Design review of the part built by this model. Coordinates are the model's own, in mm. A direction names the side the tool comes from. Give positions to 0.01 mm unless a question says otherwise; leave off trailing zeros. Write each loop counter-clockwise with the first axis right and the second up, starting at its lowest first coordinate (ties: lowest second). Pieces come first, ordered by that corner, then holes.
```python
from build123d import *

# Parameters (mm, degrees)
F0_W      = 400
F0_H      = 500
F1_DEPTH  = 2
F2_W      = 400
F2_H      = 500
F2_W_2    = 396
F2_H_2    = 496
F3_DEPTH  = 248
F5_DEPTH  = 500
F7_DEPTH  = 20
F8_R      = 5
F10_R     = 4
F11_DEPTH = 25
F12_R     = 5


with BuildPart() as f1:
    # F0 (on Top) → F1 (new body)
    with BuildSketch(Plane.XY):
        Rectangle(F0_W, F0_H)
    extrude(amount=F1_DEPTH)

    # F2 (on face) → F3 (join)
    with BuildSketch(Plane.XY.offset(2)):
        Rectangle(F2_W, F2_H)
        Rectangle(F2_W_2, F2_H_2, mode=Mode.SUBTRACT)
    extrude(amount=F3_DEPTH)

    # F4 (on face) → F5 (join)
    with BuildSketch(Plane.XZ.offset(250)):
        Polygon((215, 250), (200, 250), (200, 235), (202, 235), (202, 248), (215, 248), align=None)
        Polygon((-200, 235), (-200, 250), (-215, 250), (-215, 248), (-202, 248), (-202, 235), align=None)
    extrude(amount=-F5_DEPTH)

    # F6 (on Right) → F7 (join, symmetric)
    with BuildSketch(Plane.YZ):
        with BuildLine():
            Line((-256, 260), (-280, 260))
            Line((-280, 260), (-280, 256))
            Line((-280, 256), (-256, 256))
            ThreePointArc((-256, 256), (-254.585786, 255.414214), (-254, 254))
            Line((-254, 254), (-254, 230))
            Line((-254, 230), (-250, 230))
            Line((-250, 230), (-250, 254))
            ThreePointArc((-250, 254), (-251.757359, 258.242641), (-256, 260))
        make_face()
    extrude(amount=F7_DEPTH, both=True)

    # F8
    f8_edges = [f1.edges().sort_by_distance(p)[0] for p in [
        (20, -280, 258),
        (-20, -280, 258),
    ]]
    fillet(f8_edges, radius=F8_R)

    # F10 (on face) → F11 (cut)
    with BuildSketch(Plane.XY.offset(260)):
        with Locations((0, -270)):
            Circle(F10_R)
    extrude(amount=-F11_DEPTH, mode=Mode.SUBTRACT)

    # F12
    f12_edges = [f1.edges().sort_by_distance(p)[0] for p in [
        (20, -252, 230),
        (-20, -252, 230),
    ]]
    fillet(f12_edges, radius=F12_R)


solid = f1.part
```
(1) Consider section C-C, the plane x = 47. Give the boundary of the cut face in (y, z), then the cut area to 3 significant figures.
Resolved:
outline: (-250, 0) - (250, 0) - (250, 250) - (248, 250) - (248, 2) - (-248, 2) - (-248, 250) - (-250, 250) - close
area: 1,990 mm2
(2) Consider section A-A, the plane z = 98. Give the boundary of the cut face in (x, y).
Resolved:
outline: (-200, -250) - (200, -250) - (200, 250) - (-200, 250) - close; hole (-198, -248) - (198, -248) - (198, 248) - (-198, 248) - close
(3) To check wall thickness, follow L1, parallel to X at y = 111.5, z = 230; L2, parallel to X at y = 184, z = 239; L3, parallel to Y at x = 16, z = 43. State the ranges of each line that lie inside material, in increasing order.
Resolved:
L1: x = -200 to -198, 198 to 200
L2: x = -202 to -198, 198 to 202
L3: y = -250 to -248, 248 to 250
(4) Consider section B-B, the plane y = -165. Give the boundary of the cut face in (x, z).
Resolved:
outline: (-215, 248) - (-202, 248) - (-202, 235) - (-200, 235) - (-200, 0) - (200, 0) - (200, 235) - (202, 235) - (202, 248) - (215, 248) - (215, 250) - (198, 250) - (198, 2) - (-198, 2) - (-198, 250) - (-215, 250) - close
(5) Tool access review of faces 5 (the face through (-200, -3, 116)), 6 (the face through (200, -3, 116)), 7 (the face through (-198, -3, 124)): name each direction out of +Z, -Z, +X, -X, +Y, -Y from which nothing blocks a thin tool from reaching the whole face with its end or side.
Resolved:
face 5: -Z, -X, +Y, -Y
face 6: -Z, +X, +Y, -Y
face 7: +Z
(6) Clearance check with flat-ended pins moving along their axes: P1, Ø1, axis at x = -201.5, y = 53.5, coming from the -Z side; P2, Ø4, axis at x = 205.5, y = -66.5, coming from the -Z side; P3, Ø1, axis at x = -78.5, y = 53, coming from the +Z side. State where each tip first meets the part, or that it passes through.
Resolved:
P1: stops at z = 235
P2: stops at z = 248
P3: stops at z = 2
(7) Mouldability with a two-part tool opening along Y and no side actions: class faces 1 (the face through (-3, 3, 2)), 2 (the face through (-3, 4, 0)), 3 (the face through (-3, 250, 127)), 4 (the face through (0, -254, 242)) as pulls with the +Y half, pulls with the -Y half, needs draft (parallel to the pull), parting line crosses it, or undercut.
Resolved:
face 1: undercut
face 2: needs draft
face 3: pulls with the +Y half
face 4: pulls with the -Y half
